CAD build for the part. Positions are in the model's coordinates, mm. A direction names the side the tool comes from. Coordinates: 2 decimals unless noted, no trailing zeros. Write each loop counter-clockwise with the first axis right and the second up, starting at its lowest first coordinate (ties: lowest second). Pieces come first, ordered by that corner, then holes.
```python
from build123d import *

# Parameters (mm, degrees)
F1_W     = 47.4542081356
F1_H     = 32.0040024817
F2_DEPTH = 6.35
F0_W     = 63.5
F0_H     = 120.65
F3_DEPTH = 38.1
F4_T     = -2.54
F5_DEPTH = 2.54
F6_W     = 9.9322763272
F6_H     = 13.2430342492
F7_DEPTH = 44.451


with BuildPart() as f2:
    # F1 (on Top) → F2 (new body)
    with BuildSketch(Plane.XY):
        Rectangle(F1_W, F1_H)
    extrude(amount=-F2_DEPTH)

    # F0 (on Top) → F3 (join)
    with BuildSketch(Plane.XY):
        Rectangle(F0_W, F0_H)
    extrude(amount=F3_DEPTH)

    # F4
    f4_openings = [f2.faces().sort_by_distance(p)[0] for p in [
        (0, 0, 38.1),
    ]]
    offset(amount=F4_T, openings=f4_openings, kind=Kind.INTERSECTION)

    # F5 (cut): a face of the model
    f5_faces = [f2.faces().sort_by_distance(p)[0] for p in [
        (0, 60.325, 19.05),
    ]]
    extrude(f5_faces, amount=-F5_DEPTH, mode=Mode.SUBTRACT)

    # F6 (on face) → F7 (cut, through all)
    with BuildSketch(Plane(origin=(0, 0, -6.35), x_dir=(1, 0, 0), z_dir=(0, 0, -1))):
        with Locations((11.5876549389, 3.8625515299)):
            Rectangle(F6_W, F6_H)
        with Locations((-10.7599645853, 4.1384489741)):
            Rectangle(F6_W, F6_H)
    extrude(amount=-F7_DEPTH, mode=Mode.SUBTRACT)


solid = f2.part
```
Item 1: Saw through at A-A, the plane x = -11.5. Write the cut outline in (y, z) (3 decimals).
Item 2: Flat gauge pins, fed straight in: pin 1 Ø1.9 at (y, z) = (0, -2.5) entering from +X; pin 2 Ø0.8 at (x, z) = (10.5, -5.5) entering from -Y; pin 3 Ø3 at (x, y) = (-24.5, -27.5) entering from +Z. Where does each tip first touch, or does it go through?
Item 3: Saw through at D-D, the plane x = 18.5. Write the cut outline in (y, z) (3 decimals).
Item 4: Two-plate mould, pull along Y, no slides. Class faces 1 (the flat face through (-3, 57.785, 2)), 2 (the flat face through (-11, 2.483, -5)), 3 (the flat face through (0, -16.002, -3)): +Y half, -Y half, draft (parallel to the pull), parting line (faces both ways), or undercut.
Item 5: Wall check: line 1 along X through (y, z) = (1.5, 20.5); line 2 along Y through (x, z) = (11, 5.5) (3 decimals); line 3 along Z through (x, y) = (-2, -40.5). Give the ranges that are in metal, low to high.
Item 6: Saw through at B-B, the plane y = 5. Write the cut outline in (x, z), and give its area (3 significant figures).
Item 7: Which spindle directions (+Z, -Z, +X, -X, +Y, -Y) get a long thin tool onto all of the face, cutting with end or side? Do faces 4 (the flat face through (29.21, -1, 20)), 5 (the flat face through (23.727, 0, -3)), 6 (the flat face through (6.622, -4, -5)). Say none if no direction does.
Item 8: Saw through at C-C, the plane z = 25.5. Write the cut outline in (x, y) (3 decimals), and give its area (3 significant figures).
Working result:
1. outline: (-60.325, 0) - (-16.002, 0) - (-16.002, -6.35) - (-10.76, -6.35) - (-10.76, -3.81) - (-13.462, -3.81) - (-13.462, 2.54) - (-57.785, 2.54) - (-57.785, 38.1) - (-60.325, 38.1) - close; (2.483, -6.35) - (16.002, -6.35) - (16.002, 0) - (57.785, 0) - (57.785, 2.54) - (13.462, 2.54) - (13.462, -3.81) - (2.483, -3.81) - close
2. pin 1: stops at x = 23.73
2. pin 2: stops at y = -16
2. pin 3: stops at z = 2.54
3. outline: (-60.325, 0) - (-16.002, 0) - (-16.002, -6.35) - (16.002, -6.35) - (16.002, 0) - (57.785, 0) - (57.785, 2.54) - (13.462, 2.54) - (13.462, -3.81) - (-13.462, -3.81) - (-13.462, 2.54) - (-57.785, 2.54) - (-57.785, 38.1) - (-60.325, 38.1) - close
4. face 1: +Y half
4. face 2: undercut
4. face 3: -Y half
5. line 1: x = -31.75 to -29.21, 29.21 to 31.75
5. line 2: y = -60.325 to -57.785
5. line 3: z = 0 to 2.54
6. outline: (-31.75, 0) - (-23.73, 0) - (-23.73, -6.35) - (23.73, -6.35) - (23.73, 0) - (31.75, 0) - (31.75, 38.1) - (29.21, 38.1) - (29.21, 2.54) - (21.19, 2.54) - (21.19, -3.81) - (-21.19, -3.81) - (-21.19, 2.54) - (-29.21, 2.54) - (-29.21, 38.1) - (-31.75, 38.1) - close
6. area: 374 mm2
7. face 4: +Z, +Y
7. face 5: -Z, +X, +Y, -Y
7. face 6: +Z, -Z
8. outline: (-31.75, -60.325) - (31.75, -60.325) - (31.75, 57.785) - (29.21, 57.785) - (29.21, -57.785) - (-29.21, -57.785) - (-29.21, 57.785) - (-31.75, 57.785) - close
8. area: 748 mm2
